Geometry: see drawing. Coordinates: mm, zero at the bounding-box minimum. Give positions to 0.01 mm unless a question says otherwise; leave off trailing zeros. Write each loop counter-clockwise with the first axis right and the second up, starting at its lowest first coordinate (ties: lowest second). Pieces come first, ordered by that corner, then holes.
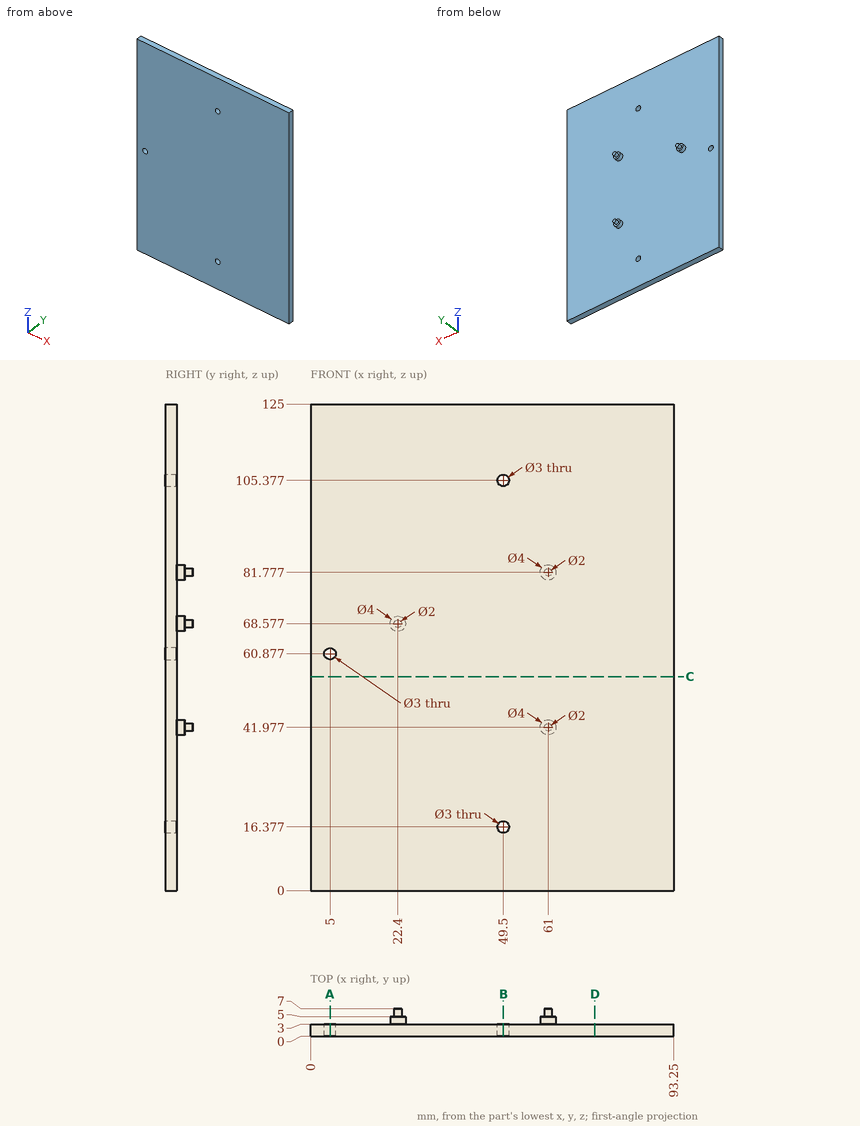
Q1. Section D-D, the plane x = 73. Return the cut outline in (y, z).
Q2. Material intervals for line 1 along Z through (x, y) = (49, 1.25); line 2 along Y through (x, z) = (83, 68); line 3 along Z through (x, y) = (59.5, 4) (1 decimal), sorted ascending.
Q3. Section A-A, the plane x = 5. Return the cut outline in (y, z), then the cut area to 3 significant figures.
Q4. Section C-C, the plane z = 55. Return the cut outline in (x, y), then the cut area to 3 significant figures.
Q5. Section B-B, the plane x = 49.5. Return the cut outline in (y, z), then the cut area to 3 significant figures.
Q6. Pin query (flat end, axial travel): pin 1 (12 mm diameter, centred on x = 36, z = 24.5, fed in from +Y); pin 2 (2.5 mm diameter, centred on x = 49.5, z = 105.38, fed in from +Y). Return the tip coordinate at first contact, or that it passes through.
Solutions:
1. outline: (0, 0) - (3, 0) - (3, 125) - (0, 125) - close
2. line 1: z = 0 to 14.96, 17.79 to 103.96, 106.79 to 125
2. line 2: y = 0 to 3
2. line 3: z = 40.7 to 43.3, 80.5 to 83.1
3. outline: (0, 0) - (3, 0) - (3, 59.38) - (0, 59.38) - close; (0, 62.38) - (3, 62.38) - (3, 125) - (0, 125) - close
3. area: 366 mm2
4. outline: (0, 0) - (93.25, 0) - (93.25, 3) - (0, 3) - close
4. area: 280 mm2
5. outline: (0, 0) - (3, 0) - (3, 14.88) - (0, 14.88) - close; (0, 17.88) - (3, 17.88) - (3, 103.88) - (0, 103.88) - close; (0, 106.88) - (3, 106.88) - (3, 125) - (0, 125) - close
5. area: 357 mm2
6. pin 1: stops at y = 3
6. pin 2: passes through
